Geometry: final body of the model. Coordinates: model frame, mm. Round coordinates to 2 decimals unless told otherwise and drop trailing zeros. Order: outer loops, then holes, each group sorted by start corner. A loop starts at its lowest first (then second) coordinate and runs counter-clockwise, first axis right, second up. Notation, with made-up numbers: M 71,82.25 L 100,82.25 A18 ccw 100,110.25 Z; hole C 10.5,-37 d2. An arc over 180 degrees is marked long. Put each result on its own line as item: value. Start each with the question number.
1) Material intervals for probe 1 along Y at (x, z) = (9.5, 0.7); probe 2 along X at (y, z) = (-28.5, 1.1); probe 3 along X at (y, z) = (-22.5, 0), sorted ascending. Write a range as [from, to].
2) First-contact query: P1, Ø1, axis at y = -61.5, z = 1, coming from the -X side; P2, Ø1.5, axis at y = -98, z = 0.5, coming from the +X side. Flat tips, straight axial feed; report the tip coordinate or a pass-through.
3) Section C-C, the plane x = 0.5. Return loops of the section in (y, z), then the cut area to 3 significant figures.
4) Section A-A, the plane z = 0.85. Return loops of the section in (x, y).
5) Draft query along X for faces 1 (the cylindrical face through (-66.7, 54.4, 1)), 2 (the cylindrical face through (-25.843, 39.245, 0.972)), 3 (the cylindrical face through (-33.23, 26.03, 0.97)), 4 (the cylindrical face through (6.241, 3.802, 0.972)). Return one class per face: pulls with the +X half, pulls with the -X half, needs draft (parallel to the pull), parting line crosses it, or undercut.
6) Section B-B, the plane y = 38. Return loops of the section in (x, z) (3 decimals), then the cut area to 3 significant figures.
from build123d import *

# Parameters (mm, degrees)
SKETCH_1_R          = 1.5
SKETCH_1_R_2        = 1
EXTRUDE_1_DEPTH     = 2
SCALE_1_SCALE       = 2
SKETCH_3_R          = 1.627142949
SKETCH_3_R_2        = 4.234260579
SKETCH_3_R_3        = 3
EXTRUDE_3_DEPTH     = 4
SKETCH_2_R          = 3
CUT_EXTRUDE_1_DEPTH = 4


with BuildPart() as part:
    # 草图1 → 凸台-拉伸1 (new body)
    with BuildSketch(Plane.XY):
        with BuildLine():
            Line((107.302513423, -106.329977447), (101.737876551, -109.126595767))
            ThreePointArc((101.737876551, -109.126595767), (100.241041238, -109.247857431), (99.081776454, -108.293223729))
            ThreePointArc((99.081776454, -108.293223729), (96.076157143, -102.895430459), (92.952174798, -97.565265927))
            ThreePointArc((92.952174798, -97.565265927), (92.67119221, -96.396525563), (93.110928625, -95.277804356))
            ThreePointArc((93.110928625, -95.277804356), (93.386262354, -90.634283432), (89.082079375, -88.870167754))
            ThreePointArc((89.082079375, -88.870167754), (87.883298953, -88.781676215), (86.951761021, -88.02197737))
            ThreePointArc((86.951761021, -88.02197737), (63.249240179, -56.927091802), (35.446375502, -29.437055089))
            ThreePointArc((35.446375502, -29.437055089), (34.93756912, -29.118601809), (34.357184804, -28.965466337))
            ThreePointArc((34.357184804, -28.965466337), (31.162596189, -27.612410648), (29.250996223, -24.717252331))
            ThreePointArc((29.250996223, -24.717252331), (28.99483955, -24.174407799), (28.589143834, -23.732019493))
            ThreePointArc((28.589143834, -23.732019493), (13.863721442, -12.651321704), (-1.558710581, -2.56328331))
            ThreePointArc((-1.558710581, -2.56328331), (-2.630799159, 1.441837641), (1.322046154, 2.692989782))
            ThreePointArc((1.322046154, 2.692989782), (17.996215952, -6.326789823), (33.906457747, -16.634484455))
            ThreePointArc((33.906457747, -16.634484455), (34.447529327, -16.904338105), (35.04451896, -17.000165164))
            ThreePointArc((35.04451896, -17.000165164), (38.553058948, -18.165150249), (40.712715331, -21.16563811))
            ThreePointArc((40.712715331, -21.16563811), (40.982462328, -21.706762868), (41.401593445, -22.142547854))
            ThreePointArc((41.401593445, -22.142547854), (79.427798672, -58.499548545), (108.618618094, -102.268485529))
            ThreePointArc((108.618618094, -102.268485529), (108.809267395, -104.574248701), (107.302513423, -106.329977447))
        make_face()
        Circle(SKETCH_1_R, mode=Mode.SUBTRACT)
        with Locations((105.955364791, -103.64945687)):
            Circle(SKETCH_1_R_2, mode=Mode.SUBTRACT)
        with Locations((101.955364791, -106.64945687)):
            Circle(SKETCH_1_R_2, mode=Mode.SUBTRACT)
        with Locations((35, -23)):
            Circle(SKETCH_1_R, mode=Mode.SUBTRACT)
    extrude(amount=EXTRUDE_1_DEPTH)


with BuildPart() as part_1:
    # 缩放比例1: scaled about (61.378569751, -51.627856738, 1)
    add(part.part.scale(SCALE_1_SCALE).moved(Location((-61.378569751, 51.627856738, -1))))

    # 草图3 → 凸台-拉伸3 (add)
    # profile 1 of 8: a face of its own
    with BuildSketch(Plane(origin=(0, 0, -1), x_dir=(-1, 0, 0), z_dir=(0, 0, -1))):
        with Locations((58.543077077, 54.655425944)):
            Circle(SKETCH_3_R)
    # profile 2 of 8: a face of its own
    with BuildSketch(Plane(origin=(0, 0, -1), x_dir=(-1, 0, 0), z_dir=(0, 0, -1))):
        with Locations((61.20941419, 50.866420573)):
            Circle(SKETCH_3_R_2)
        with Locations((61.378569751, 51.627856738)):
            Circle(SKETCH_3_R_3, mode=Mode.SUBTRACT)
    # profile 3 of 8: a face of its own
    with BuildSketch(Plane(origin=(0, 0, -1), x_dir=(-1, 0, 0), z_dir=(0, 0, -1))):
        with Locations((58.543077077, 54.655425944)):
            Circle(SKETCH_3_R)
    # profile 4 of 8: a face of its own
    with BuildSketch(Plane(origin=(0, 0, -1), x_dir=(-1, 0, 0), z_dir=(0, 0, -1))):
        with Locations((58.543077077, 54.655425944)):
            Circle(SKETCH_3_R)
    # profile 5 of 8: a face of its own
    with BuildSketch(Plane(origin=(0, 0, -1), x_dir=(-1, 0, 0), z_dir=(0, 0, -1))):
        with Locations((61.20941419, 50.866420573)):
            Circle(SKETCH_3_R_2)
        with Locations((61.378569751, 51.627856738)):
            Circle(SKETCH_3_R_3, mode=Mode.SUBTRACT)
    # profile 6 of 8: a face of its own
    with BuildSketch(Plane(origin=(0, 0, -1), x_dir=(-1, 0, 0), z_dir=(0, 0, -1))):
        with Locations((61.378569751, 51.627856738)):
            Circle(SKETCH_3_R_3)
    # profile 7 of 8: a face of its own
    with BuildSketch(Plane(origin=(0, 0, -1), x_dir=(-1, 0, 0), z_dir=(0, 0, -1))):
        with Locations((58.543077077, 54.655425944)):
            Circle(SKETCH_3_R)
    # profile 8 of 8: a face of its own
    with BuildSketch(Plane(origin=(0, 0, -1), x_dir=(-1, 0, 0), z_dir=(0, 0, -1))):
        with Locations((61.378569751, 51.627856738)):
            Circle(SKETCH_3_R_3)
    extrude(amount=-EXTRUDE_3_DEPTH)

    # 草图2 → 切除-拉伸1 (cut)
    with BuildSketch(Plane.XY.offset(3)):
        with Locations((-57.967630724, 49.966726496)):
            Circle(SKETCH_2_R)
    extrude(amount=-CUT_EXTRUDE_1_DEPTH, mode=Mode.SUBTRACT)


solid = part_1.part
Result sheet:
1. probe 1: y = [-7.23, 2.76], [8.5, 17.6]
1. probe 2: x = [32.88, 63.09]
1. probe 3: x = [26.55, 56.76]
2. P1: stops at x = 64.04
2. P2: stops at x = 123.07
3. outline: M -3.21,-1 L 22.48,-1 L 22.48,3 L -3.21,3 Z
3. area: 103 mm2
4. outline: M -64.5,46.5 A560 cw -4.2,4.16 A4 cw -2.88,2.19 A12 ccw 7.34,-6.3 A4 cw 9.51,-7.25 A560 cw 112.52,-124.42 A4 ccw 116.79,-126.11 A8 cw 124.84,-138.93 A4 ccw 124.53,-143.5 A560 cw 136.78,-164.96 A4 ccw 142.1,-166.63 L 153.23,-161.03 A6 ccw 155.86,-152.91 A480 ccw 21.42,7.34 A4 cw 20.05,9.3 A12 ccw 8.71,17.63 A4 cw 6.43,18.36 A480 ccw -58.73,57.01 A6 ccw Z; hole C -57.97,49.97 d6; hole C 8.62,5.63 d6; hole C 142.53,-161.67 d4; hole C 150.53,-155.67 d4
5. face 1: parting line crosses it
5. face 2: pulls with the +X half
5. face 3: pulls with the -X half
5. face 4: undercut
6. outline: M -50.955,-1 L -23.751,-1 L -23.751,3 L -50.955,3 Z
6. area: 109 mm2
